Input: dimensioned drawing with shaded views. Units: mm. Origin: part minimum x, y, z. A direction names the side the tool comes from. Give positions to 0.01 mm unless a question says otherwise; leave off trailing zeros. Loops run counter-clockwise (first coordinate to the right, second up) from the corner with the lowest first, then second, coordinate; pieces in that order, holes last. Notation, with made-up numbers: (-6, 65.5) -> (26, 65.5) arc R25 cw to (26, 104.5) -> close; hole circle Ø2 at (76.5, 34.5). An arc over 180 degrees is marked (long way). Answer as a JSON object with one key per item and string values.
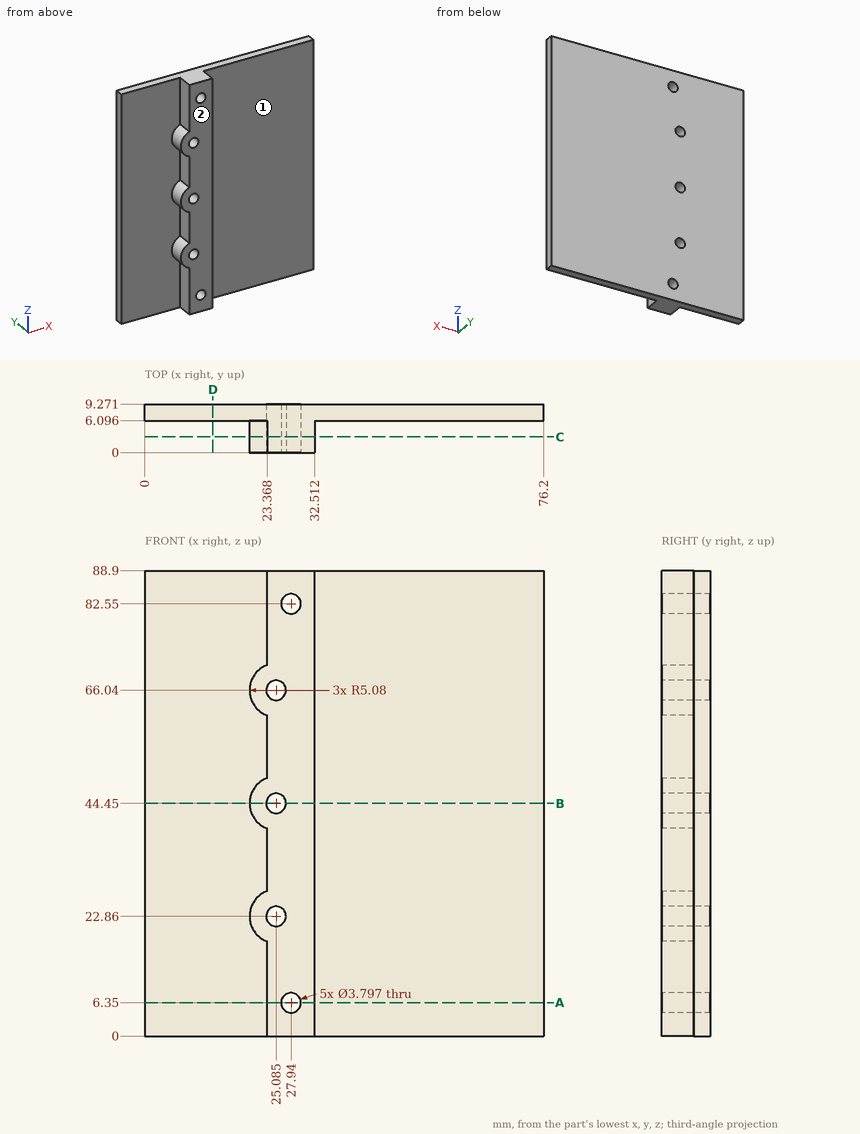
Q1. Section C-C, the plane y = 3. Give the number of separate pieces and of enclosed holes in the cut face.
Evaluation:
{"separate pieces": "1", "enclosed holes": "5"}
Q2. Access query for the marked faces 1 and 2. Directions: +Z, -Z, +X, -X, +Y, -Y. A direction counts if a zero-diameter tool reaches every point of the face in a straight line with its end or side. Return the directions, or none.
Evaluation:
{"face 1": "+Z, -Z, +X, -Y", "face 2": "+Z, -Z, +X, -X, -Y"}
Q3. Section A-A, the plane z = 6.35. Return the cut outline in (x, y).
Evaluation:
{"outline": "(0, 6.1) -> (23.37, 6.1) -> (23.37, 0) -> (26.04, 0) -> (26.04, 9.27) -> (0, 9.27) -> close; (29.84, 0) -> (32.51, 0) -> (32.51, 6.1) -> (76.2, 6.1) -> (76.2, 9.27) -> (29.84, 9.27) -> close"}
Q4. Ray query, line 1 along X through (y, z) = (5, 44.45) (1 decimal); line 2 along Z through (x, y) = (26, 1); line 3 along Z through (x, y) = (21, 2.75). Return the intervals inside material, ascending.
Evaluation:
{"line 1": "x = 20 to 23.2, 27 to 32.5", "line 2": "z = 0 to 21.2, 24.52 to 42.79, 46.11 to 64.38, 67.7 to 88.9", "line 3": "z = 19.84 to 25.88, 41.43 to 47.47, 63.02 to 69.06"}
Q5. Section D-D, the plane x = 13. Return the cut outline in (y, z).
Evaluation:
{"outline": "(6.1, 0) -> (9.27, 0) -> (9.27, 88.9) -> (6.1, 88.9) -> close"}
Q6. Section B-B, the plane z = 44.45. Return the cut outline in (x, y) (1 decimal), then the cut area to 3 significant figures.
Evaluation:
{"outline": "(0, 6.1) -> (20, 6.1) -> (20, 0) -> (23.2, 0) -> (23.2, 9.3) -> (0, 9.3) -> close; (27, 0) -> (32.5, 0) -> (32.5, 6.1) -> (76.2, 6.1) -> (76.2, 9.3) -> (27, 9.3) -> close", "area": "283 mm2"}
Q7. Pin query (flat end, axial travel): pin 1 (5 mm diameter, centred on y = 3.5, z = 55, fed in from -X); pin 2 (11.5 mm diameter, centred on x = 15, z = 33.5, fed in from -Y); pin 3 (4 mm diameter, centred on y = 1.5, z = 47, fed in from -X) (1 decimal). Return the tip coordinate at first contact, or that it passes through.
Evaluation:
{"pin 1": "stops at x = 23.37", "pin 2": "stops at y = 6.1", "pin 3": "stops at x = 20"}
